```python
from build123d import *

# Parameters (mm, degrees)
BOSS_EXTRUDE1_DEPTH = 9.6
SKETCH2_W           = 28
SKETCH2_H           = 13
BOSS_EXTRUDE2_DEPTH = 0.8
BOSS_EXTRUDE3_DEPTH = 5
SKETCH4_R           = 2
BOSS_EXTRUDE4_DEPTH = 0.1
DOME1_FACE_RADIUS   = 2
DOME1_HEIGHT        = 0.8


with BuildPart() as part:
    # Sketch1 → Boss-Extrude1 (new body)
    with BuildSketch(Plane.XY):
        Polygon((-16.122641509, -15.877358491), (-12.122641509, -15.877358491), (-12.122641509, -6.877358491), (7.877358491, -6.877358491), (7.877358491, -15.877358491), (11.877358491, -15.877358491), (11.877358491, -2.877358491), (-16.122641509, -2.877358491), align=None)
    extrude(amount=BOSS_EXTRUDE1_DEPTH)

    # Sketch2 → Boss-Extrude2 (add)
    with BuildSketch(Plane.XY.offset(9.6)):
        with Locations((-2.122641509, -9.377358491)):
            Rectangle(SKETCH2_W, SKETCH2_H)
    extrude(amount=BOSS_EXTRUDE2_DEPTH)

    # Sketch3 → Boss-Extrude3 (add)
    with BuildSketch(Plane.XZ.offset(15.877358491)):
        Polygon((-4.096861334, 10.4), (3.877358491, 10.4), (3.877358491, 17.4), (-2.122641509, 17.4), (-2.122641509, 13.817479277), (-4.096861334, 13.817479277), align=None)
        Polygon((-12.122641509, 17.4), (3.119119142, 20.087533636), (2.9802006, 20.875379839), (-12.922641509, 18.071279705), (-12.922641509, 13.961837911), (-12.922641509, 10.4), (-12.122641509, 10.4), (-12.122641509, 12.7), (-10.384503435, 12.7), (-10.384503435, 13.9), (-12.122641509, 13.9), align=None)
    extrude(amount=-BOSS_EXTRUDE3_DEPTH)

    # Sketch4 → Boss-Extrude4 (add)
    with BuildSketch(Plane(origin=(-3.480036158, 0, 19.736265797), x_dir=(0.9848077530122085, 0, 0.17364817766692794), z_dir=(-0.17364817766692794, 0, 0.9848077530122085))):
        with Locations((3.559896323, -13.377358491)):
            Circle(SKETCH4_R)
    extrude(amount=BOSS_EXTRUDE4_DEPTH)

    # Dome1: a dome of height H over a round flat face of radius A is a cap of a sphere of radius (A * A + H * H) / (2 * H)
    dome1_r = (DOME1_FACE_RADIUS * DOME1_FACE_RADIUS + DOME1_HEIGHT * DOME1_HEIGHT) / (2 * DOME1_HEIGHT)
    dome1_base = Plane((0.008412523, -13.377358491, 20.452916081), z_dir=(-0.173648177667, 0, 0.984807753012))
    with Locations(dome1_base.offset(DOME1_HEIGHT - dome1_r)):
        dome1_ball = Sphere(dome1_r, mode=Mode.PRIVATE)
    add(split(dome1_ball, bisect_by=dome1_base, keep=Keep.TOP, mode=Mode.PRIVATE))


solid = part.part
```
Geometry check sheet. Reference: the model listing, model coordinates, mm. A direction names the side the tool comes from. Round coordinates to 2 decimals unless told otherwise and drop trailing zeros. Order: outer loops, then holes, each group sorted by start corner. A loop starts at its lowest first (then second) coordinate and runs counter-clockwise, first axis right, second up. Notation, with made-up numbers: (80, -21.5) - (103, -21.5) arc R25 cw to (103, 5.5) - close; hole circle Ø1 at (-10, -11.5). An arc over 180 degrees is marked (long way). Use a Markdown table: item, result. Add a question column.
(1) Material ranges on line 1 along X through (y, z) = (-10, 2); line 2 along X through (y, z) = (-14.5, 14); line 3 along Y through (x, z) = (-11.75, 13), recorded low to high. Write a range as [from, to].
(2) Release check for a two-part mould opening along X. For faces 1 (the flat face through (-2, -2.877, 5)), 2 (the flat face through (3.877, -13, 14)), 3 (the flat face through (-11, -13, 12.7)) record: pulls with the +X half, pulls with the -X half, needs draft (parallel to the pull), parting line crosses it, or undercut.
(3) Sectioned sample at B-B, the plane y = -9.25. Enter the section's corners in (x, z).
(4) Sectioned sample at D-D, the plane z = 6.75. Enter the section's corners in (x, y).
(5) Depth check by flat-ended pin: pin 1 (5.5 mm diameter, centred on x = -0.5, y = -12.5, fed in from +Z); pin 2 (3 mm diameter, centred on x = 1.5, z = 3, fed in from -Y); pin 3 (1 mm diameter, centred on y = -14, z = 13.5, fed in from +X); pin 4 (5 mm diameter, centred on x = -3.5, z = 13.5, fed in from +Y). Enter the tip coordinate at first touch or a pass-through.
(6) Tool access check on faces 4 (the flat face through (-4.608, -13.412, 18.725)), 5 (the flat face through (-12.123, -13, 12)), 6 (the flat face through (7.877, -11, 5)), 7 (the flat face through (0, -10.877, 14)). Record the directions out of +Z, -Z, +X, -X, +Y, -Y that give a thin tool (end or side, any length) a straight path to the whole face; none if there is none.
(7) Sectioned sample at C-C, the plane x = -6. Enter the section's corners in (y, z).
(8) Sectioned sample at A-A, the plane z = 14.5. Enter the section's corners in (x, y), and give its area (3 significant figures).
Answers below:
| question | item | result |
|---|---|---|
| 1 | line 1 | [-16.12, -12.12], [7.88, 11.88] |
| 1 | line 2 | [-12.92, -12.12], [-2.12, 3.88] |
| 1 | line 3 | [-15.88, -10.88] |
| 2 | face 1 | needs draft |
| 2 | face 2 | pulls with the +X half |
| 2 | face 3 | undercut |
| 3 | outline | (-16.12, 0) - (-12.12, 0) - (-12.12, 9.6) - (7.88, 9.6) - (7.88, 0) - (11.88, 0) - (11.88, 10.4) - (-16.12, 10.4) - close |
| 4 | outline | (-16.12, -15.88) - (-12.12, -15.88) - (-12.12, -6.88) - (7.88, -6.88) - (7.88, -15.88) - (11.88, -15.88) - (11.88, -2.88) - (-16.12, -2.88) - close |
| 5 | pin 1 | z = 21.28 |
| 5 | pin 2 | y = -6.88 |
| 5 | pin 3 | x = 3.88 |
| 5 | pin 4 | y = -10.88 |
| 6 | face 4 | +X, +Y, -Y |
| 6 | face 5 | +Y, -Y |
| 6 | face 6 | -Z, -Y |
| 6 | face 7 | +Z, +X, -X, +Y |
| 7 | outline | (-15.88, 9.6) - (-6.88, 9.6) - (-6.88, 0) - (-2.88, 0) - (-2.88, 10.4) - (-15.88, 10.4) - close; (-15.88, 18.48) - (-10.88, 18.48) - (-10.88, 19.29) - (-15.88, 19.29) - close |
| 8 | outline | (-12.92, -15.88) - (-12.12, -15.88) - (-12.12, -10.88) - (-12.92, -10.88) - close; (-2.12, -15.88) - (3.88, -15.88) - (3.88, -10.88) - (-2.12, -10.88) - close |
| 8 | area | 34.0 mm² |
